Model file for the job. Use its own axes, mm. A direction names the side the tool comes from. Coordinates: 2 decimals unless noted, no trailing zeros. Loops run counter-clockwise (first coordinate to the right, second up) from the corner with the lowest first, then second, coordinate; pieces in that order, holes last. Notation, with made-up numbers: M -22,-37 L 19,-37 A24 ccw 19,-23 Z; hole C -14,-29.75 d4. An arc over 180 degrees is marked long. Write item = value, one per line. Start each with the question number.
from build123d import *

# Parameters (mm, degrees)
F0_R     = 40
F1_DEPTH = 2
F2_R     = 30
F2_R_2   = 28.5
F3_DEPTH = 2
F4_R     = 20
F4_R_2   = 18.5
F5_DEPTH = 4


with BuildPart() as f1:
    # F0 (on Top) → F1 (new body)
    with BuildSketch(Plane.XY):
        Circle(F0_R)
    extrude(amount=F1_DEPTH)

    # F2 (on face) → F3 (join)
    with BuildSketch(Plane.XY.offset(2)):
        Circle(F2_R)
        Circle(F2_R_2, mode=Mode.SUBTRACT)
    extrude(amount=F3_DEPTH)

    # F4 (on face) → F5 (join)
    with BuildSketch(Plane.XY.offset(2)):
        Circle(F4_R)
        Circle(F4_R_2, mode=Mode.SUBTRACT)
    extrude(amount=F5_DEPTH)


solid = f1.part
Item 1: Cut at D-D (x = 25.5). Give the cut face in (y, z), plus the area to 3 significant figures.
Item 2: Cut at C-C (y = -22). Give the cut face in (x, z).
Item 3: 3-axis set-ups, long thin cutter, end or side, ignore diameter. For faces 1 (the flat face through (-1, 1, 0)), 2 (the flat face through (5.9, 19.4, 2)): which of +Z, -Z, +X, -X, +Y, -Y reach the whole face in a straight line?
Item 4: Pin check, flat tips, straight feed: pin 1 Ø11 at (x, y) = (-6, 7.5) entering from +Z; pin 2 Ø3 at (x, z) = (-28.5, 1.5) entering from -Y; pin 3 Ø2 at (x, z) = (18.5, 1) entering from -Y. Stop position of each tip, or through.
Item 5: Pull direction X, two halves, no side cores. Call faces 3 (the flat face through (6, -18, 6)), 4 (the cylindrical face through (-29.97, 1.32, 2.99)), 5 (the cylindrical face through (26.327, -10.916, 2.986)): +X half, -X half, draft (parallel to the pull), parting line (faces both ways), or undercut.
Item 6: Cut at A-A (y = 0). Give the cut face in (x, z).
Item 7: Probe L1, parallel to Z at x = -28.5, y = -26; L2, parallel to Y at x = -14, z = 3.1; L3, parallel to Y at x = 0, z = 4.35. List the from-to ranges inside material, lowest first.
Reported:
q1.outline = M -30.82,0 L 30.82,0 L 30.82,2 L 15.8,2 L 15.8,4 L 12.73,4 L 12.73,2 L -12.73,2 L -12.73,4 L -15.8,4 L -15.8,2 L -30.82,2 Z
q1.area = 136 mm^2
q2.outline = M -33.41,0 L 33.41,0 L 33.41,2 L 20.4,2 L 20.4,4 L 18.12,4 L 18.12,2 L -18.12,2 L -18.12,4 L -20.4,4 L -20.4,2 L -33.41,2 Z
q3.face_1 = -Z, +X, -X, +Y, -Y
q3.face_2 = +Z
q4.pin_1 = 2
q4.pin_2 = -29.51
q4.pin_3 = -35.97
q5.face_3 = draft
q5.face_4 = parting line
q5.face_5 = undercut
q6.outline = M -40,0 L 40,0 L 40,2 L 30,2 L 30,4 L 28.5,4 L 28.5,2 L 20,2 L 20,6 L 18.5,6 L 18.5,2 L -18.5,2 L -18.5,6 L -20,6 L -20,2 L -28.5,2 L -28.5,4 L -30,4 L -30,2 L -40,2 Z
q7.L1 = 0 to 2
q7.L2 = -26.53 to -24.82, -14.28 to -12.09, 12.09 to 14.28, 24.82 to 26.53
q7.L3 = -20 to -18.5, 18.5 to 20
